Can you work these out from the model? Positions are in its coordinate system, mm. Give positions to 0.01 mm unless a question says otherwise; leave off trailing zeros. Loops run counter-clockwise (first coordinate to the right, second up) from the corner with the lowest first, then second, coordinate; pieces in that order, holes last. Notation, with made-up numbers: M 21.25,67 L 65.25,67 A14 cw 65.25,79 Z; hole C -9,85.5 d5. An arc over 180 degrees is marked long. Put each result on its own line as item: value. Start each with the question number.
1) For P1, Ø5, axis at x = 91, y = -162, coming from the -Z side; P2, Ø1, axis at y = -27.5, z = 131, coming from the +X side; P3, Ø17.5, axis at x = 30, y = -87.5, coming from the +Z side, each with a flat end and sliding along its axis, tell me the tip position at first contact or that it passes through.
2) Imagine slicing it at C-C (z = 173). Write out the boundary of the cut face in (x, y), then the cut area to 3 significant figures.
3) Imagine slicing it at A-A (y = -153). Write out the boundary of the cut face in (x, z) (1 decimal).
4) Imagine slicing it at B-B (y = -43). Write out the boundary of the cut face in (x, z) (1 decimal), then the cut area to 3 significant figures.
5) Imagine slicing it at D-D (z = 150). Write out the boundary of the cut face in (x, y).
6) Please list where these lines run through material, in increasing order: line 1 along Z through (x, y) = (63.5, -69); line 2 along Z through (x, y) = (63, -113); line 3 along Z through (x, y) = (61.5, -9). Write a range as from..to.
from build123d import *

# Parameters (mm, degrees)
F1_DEPTH = 190.5
F3_DEPTH = 21.9964
F4_R     = 6.35
F5_DEPTH = 68.1482
F6_D     = 6.35


with BuildPart() as f1:
    # F0 (on Front) → F1 (new body)
    with BuildSketch(Plane.XZ):
        with BuildLine():
            Line((0, 12.7), (0, 0))
            Line((0, 0), (70.8406, 0))
            Line((70.8406, 0), (176.1109, 182.333508128))
            Line((176.1109, 182.333508128), (165.8914941513, 188.2336848457))
            Line((165.8914941513, 188.2336848457), (65.8996305851, 16.8137791998))
            ThreePointArc((65.8996305851, 16.8137791998), (65.872041904, 8.5702514052), (58.7375, 12.7))
            Line((58.7375, 12.7), (0, 12.7))
        make_face()
    extrude(amount=F1_DEPTH)

    # F2 (on face) → F3 (join)
    with BuildSketch(Plane.XY.offset(12.7)):
        with BuildLine():
            ThreePointArc((25.4, -6.35), (20.9098719395, -17.1901280605), (31.75, -12.7))
            ThreePointArc((31.75, -12.7), (29.8901280605, -8.2098719395), (25.4, -6.35))
        make_face()
    extrude(amount=F3_DEPTH)

    # F4 (on face) → F5 (join)
    with BuildSketch(Plane(origin=(41.8516023858, 0, -24.4126824129), x_dir=(0, -1, 0), z_dir=(-0.8637856588, 0, 0.5038594404))):
        with Locations((12.7, 81.1343050771)):
            Circle(F4_R)
    extrude(amount=F5_DEPTH)

    # F6 (through all)
    with Locations(Plane(origin=(41.8516023858, 0, -24.4126824129), x_dir=(0, -1, 0), z_dir=(-0.8637856588, 0, 0.5038594404))):
        with Locations((12.7, 195.3795528826), (12.7, 144.5795528826), (76.2, 144.5795528826), (152.4, 144.5795528826)):
            Hole(F6_D / 2)


solid = f1.part
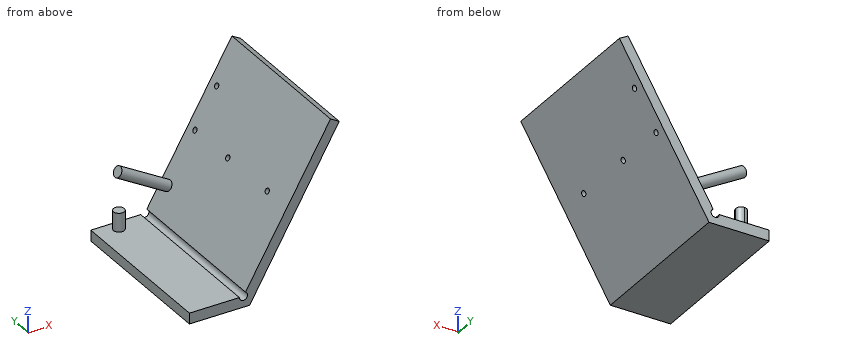
Recorded:
1. P1: z = 30.59
1. P2: x = 146.76
1. P3: z = 12.7
2. outline: M 157.01,-190.5 L 170.72,-190.5 L 170.72,0 L 157.01,0 Z
2. area: 2,610 mm²
3. outline: M 0,0 L 70.8,0 L 123.7,91.6 L 113.1,97.8 L 65.9,16.8 A4.8 cw long 58.7,12.7 L 0,12.7 Z; M 116.3,103.2 L 126.8,97 L 176.1,182.3 L 165.9,188.2 Z
4. outline: M 0,0 L 70.8,0 L 176.1,182.3 L 165.9,188.2 L 65.9,16.8 A4.8 cw long 58.7,12.7 L 0,12.7 Z
4. area: 3,340 mm²
5. outline: M 143.59,-190.5 L 157.44,-190.5 L 157.44,0 L 143.59,0 Z
6. line 1: 0..7.94
6. line 2: 0..7.96
6. line 3: 0..8.38, 52.08..64.03
